from build123d import *

# Parameters (mm, degrees)
F1_DEPTH = 388.820231


with BuildPart() as f1:
    # F0 (on Top) → F1 (new body)
    with BuildSketch(Plane.XY):
        Polygon((33.697896, -0.176251), (33.548033, 0), (0, 0), align=None)
        Polygon((0, 0), (33.548033, 0), (-94.663486, 150.786906), (-131.025478, 150.786906), align=None)
    extrude(amount=F1_DEPTH)


solid = f1.part
For this review, take the finished solid that the model builds, in its own axes (mm). Round coordinates to 2 decimals unless told otherwise and drop trailing zeros. Order: outer loops, then holes, each group sorted by start corner. A loop starts at its lowest first (then second) coordinate and runs counter-clockwise, first axis right, second up. Notation, with made-up numbers: M 10,68.25 L 64,68.25 A12 cw 64,86.25 Z; hole C -13,59 d3. An arc over 180 degrees is marked long. Write each question's results on one line, items separated by ' | '. Start each with the question number.
1. Clearance check with flat-ended pins moving along their axes: pin 1 Ø5 at (y, z) = (38.5, 115.5) entering from +X; pin 2 Ø8 at (y, z) = (111, 40) entering from +X; pin 3 Ø6 at (x, z) = (-58, 260) entering from +Y. State where each tip first meets the part, or that it passes through.
2. Add section A-A (z = 223). State the section outline as (x, y) points.
3. Add section B-B (x = -105). State the section outline as (y, z) points.
4. Add section C-C (y = 94). State the section outline as (x, z) points, then the cut area to 3 significant figures.
5. To check wall thickness, follow L1, parallel to X at y = 55, z = 263; L2, parallel to Y at x = -92.5, z = 335; L3, parallel to X at y = 37.5, z = 345. State the ranges of each line that lie inside material, in increasing order. Write a range as [from, to].
Output values:
1) pin 1: x = 2.94 | pin 2: x = -57.43 | pin 3: y = 111.2
2) outline: M -131.03,150.79 L 0,0 L 33.7,-0.18 L 33.55,0 L -94.66,150.79 Z
3) outline: M 120.84,0 L 150.79,0 L 150.79,388.82 L 120.84,388.82 Z
4) outline: M -81.68,0 L -46.38,0 L -46.38,388.82 L -81.68,388.82 Z | area: 13,700 mm^2
5) L1: [-47.79, -13.22] | L2: [106.45, 148.24] | L3: [-32.59, 1.66]
